```python
from build123d import *

# Parameters (mm, degrees)
SKETCH1_W               = 50
SKETCH1_H               = 50
BOSS_EXTRUDE1_DEPTH     = 2
SKETCH2_W               = 8.5
SKETCH2_H               = 2
SKETCH2_W_2             = 26.5
BOSS_EXTRUDE2_DEPTH     = 20
SKETCH3_W               = 2
SKETCH3_H               = 15
BOSS_EXTRUDE3_DEPTH     = 15
SKETCH5_W               = 2
SKETCH5_H               = 15
BOSS_EXTRUDE5_DEPTH     = 25
SKETCH6_W               = 8
SKETCH6_H               = 5
SKETCH6_H_2             = 10
BOSS_EXTRUDE6_DEPTH     = 2
FILLET1_R               = 10
FILLET2_R               = 10
FILLET3_R               = 5
CUT_EXTRUDE1_DEPTH      = 58.567351858
CUT_EXTRUDE1_DEPTH_BACK = 58.567351858
SKETCH7_R               = 1.65
SKETCH8_W               = 3.5
SKETCH8_H               = 6
BOSS_EXTRUDE7_DEPTH     = 8


with BuildPart() as part:
    # Sketch1 → Boss-Extrude1 (new body)
    with BuildSketch(Plane.XY):
        Rectangle(SKETCH1_W, SKETCH1_H)
    extrude(amount=BOSS_EXTRUDE1_DEPTH)

    # Sketch2 → Boss-Extrude2 (add)
    with BuildSketch(Plane(origin=(0, 0, 0), x_dir=(-1, 0, 0), z_dir=(0, 0, -1))):
        with Locations((-20.75, -24)):
            Rectangle(SKETCH2_W, SKETCH2_H)
        with Locations((11.75, -24)):
            Rectangle(SKETCH2_W_2, SKETCH2_H)
    extrude(amount=BOSS_EXTRUDE2_DEPTH)

    # Sketch3 → Boss-Extrude3 (add)
    with BuildSketch(Plane.XZ.offset(25)):
        with Locations((24, -5.5)):
            Rectangle(SKETCH3_W, SKETCH3_H)
    extrude(amount=BOSS_EXTRUDE3_DEPTH)

    # Sketch5 → Boss-Extrude5 (add)
    with BuildSketch(Plane(origin=(0, 0, 0), x_dir=(-1, 0, 0), z_dir=(0, 0, -1))):
        with Locations((-20.5, 5.5)):
            Rectangle(SKETCH5_W, SKETCH5_H)
        with Locations((22, 5.5)):
            Rectangle(SKETCH5_W, SKETCH5_H)
    extrude(amount=BOSS_EXTRUDE5_DEPTH)

    # Sketch6 → Boss-Extrude6 (add)
    with BuildSketch(Plane(origin=(0, 0, 0), x_dir=(-1, 0, 0), z_dir=(0, 0, -1))):
        with Locations((-29, -14)):
            Rectangle(SKETCH6_W, SKETCH6_H)
        with Locations((-29, 26)):
            Rectangle(SKETCH6_W, SKETCH6_H_2)
    extrude(amount=-BOSS_EXTRUDE6_DEPTH)

    # Fillet1
    # the kernel refuses this fillet: 10 mm, written as the material it adds along each edge
    with BuildSketch(Plane(origin=(25, 25, 0), x_dir=(-1, 0, 0), z_dir=(0, 0, 1))) as fillet1_piece_1:
        with BuildLine():
            CenterArc((9.16515139, -10), FILLET1_R, 90, 66.421821522)
            Line((0, -6), (-0.183303028, -5.92))
            ThreePointArc((-0.183303028, -5.92), (-0.2, -3), (-0.2, 0))
            Line((-0.2, 0), (0, 0.2))
            Line((0, 0.2), (9.16515139, 0.2))
            Line((9.16515139, 0.2), (9.16515139, 0))
        make_face()
    extrude(amount=2)

    # Fillet2
    # the kernel refuses this fillet: 10 mm, written as the material it adds along each edge
    with BuildSketch(Plane(origin=(25, 21, 0), x_dir=(0, -1, 0), z_dir=(0, 0, 1))) as fillet2_piece_1:
        with BuildLine():
            CenterArc((9.797958971, 10), FILLET2_R, 191.536959033, 78.463040967)
            Line((0, 8), (-0.195959179, 7.96))
            ThreePointArc((-0.195959179, 7.96), (-0.2, 4), (-0.2, 0))
            Line((-0.2, 0), (0, -0.2))
            Line((0, -0.2), (9.797958971, -0.2))
            Line((9.797958971, -0.2), (9.797958971, 0))
        make_face()
    extrude(amount=2)

    # Fillet3
    fillet3_edges = [part.edges().sort_by_distance(p)[0] for p in [
        (25, -16.5, 1),
        (25, -11.5, 1),
    ]]
    fillet(fillet3_edges, radius=FILLET3_R)

    # Sketch7 → Cut-Extrude1 (cut, two sides: drawn at the far end of the back side and taken through both)
    with BuildSketch(Plane(origin=(0, 0, 0), x_dir=(-1, 0, 0), z_dir=(0, 0, -1)).offset(-CUT_EXTRUDE1_DEPTH_BACK)):
        with Locations((-29.35, -14)):
            Circle(SKETCH7_R)
        with Locations((-29.35, 26)):
            Circle(SKETCH7_R)
    extrude(amount=CUT_EXTRUDE1_DEPTH + CUT_EXTRUDE1_DEPTH_BACK, mode=Mode.SUBTRACT)

    # Sketch8 → Boss-Extrude7 (add)
    with BuildSketch(Plane(origin=(0, 0, 0), x_dir=(-1, 0, 0), z_dir=(0, 0, -1))):
        with Locations((23.25, -11)):
            Rectangle(SKETCH8_W, SKETCH8_H)
    extrude(amount=BOSS_EXTRUDE7_DEPTH)


solid = part.part
```
Read the model definition and answer for the solid it produces. Units are mm, in the model's axes. A direction names the side the tool comes from. Coordinates: 2 decimals unless noted, no trailing zeros. Write each loop counter-clockwise with the first axis right and the second up, starting at its lowest first coordinate (ties: lowest second). Pieces come first, ordered by that corner, then holes. Notation, with made-up numbers: (28, 21.25) -> (71, 21.25) arc R28 cw to (71, 52.25) -> close; hole circle Ø9 at (-33.5, 81.25). An arc over 180 degrees is marked (long way). Return JSON: item names as keys, results as strings.
1. A cutting plane is placed at C-C (z = -4.5). Determine the outline of the cut face in (x, y), and give its area (3 significant figures).
Found:
{"outline": "(-25, -25) -> (1.5, -25) -> (1.5, -23) -> (-25, -23) -> close; (-25, -14) -> (-21.5, -14) -> (-21.5, -8) -> (-25, -8) -> close; (-23, -2) -> (-21, -2) -> (-21, 13) -> (-23, 13) -> close; (16.5, -25) -> (23, -25) -> (23, -40) -> (25, -40) -> (25, -23) -> (16.5, -23) -> close; (19.5, -2) -> (21.5, -2) -> (21.5, 13) -> (19.5, 13) -> close", "area": "181 mm2"}
2. A cutting plane is placed at D-D (y = 26). Determine the outline of the cut face in (x, z), and give its area (3 significant figures).
Found:
{"outline": "(20.19, 0) -> (27.7, 0) -> (27.7, 2) -> (20.19, 2) -> close; (31, 0) -> (33, 0) -> (33, 2) -> (31, 2) -> close", "area": "19.0 mm2"}
3. Determine the mould class of faces 1 (the face through (25, -31, -7)), 2 (the face through (21, -2, -12)), 3 (the face through (-22, 13, -12)) for opening direction Y: pulls with the +Y half, pulls with the -Y half, needs draft (parallel to the pull), parting line crosses it, or undercut.
Found:
{"face 1": "needs draft", "face 2": "undercut", "face 3": "pulls with the +Y half"}
4. A cutting plane is placed at A-A (z = -11.5). Determine the outline of the cut face in (x, y), and give its area (3 significant figures).
Found:
{"outline": "(-25, -25) -> (1.5, -25) -> (1.5, -23) -> (-25, -23) -> close; (-23, -2) -> (-21, -2) -> (-21, 13) -> (-23, 13) -> close; (16.5, -25) -> (23, -25) -> (23, -40) -> (25, -40) -> (25, -23) -> (16.5, -23) -> close; (19.5, -2) -> (21.5, -2) -> (21.5, 13) -> (19.5, 13) -> close", "area": "160 mm2"}
5. Find the intervals of material crossed by line 1 along Y through (x, z) = (29.35, 0.75); line 2 along X through (y, z) = (-14, 1.45); line 3 along Z through (x, y) = (-18, 12), in increasing order. Write a range as from..to.
Found:
{"line 1": "-16.54..-15.65, -12.35..-11.46, 19.45..24.35, 27.65..31", "line 2": "-25..27.7, 31..33", "line 3": "0..2"}
6. A tool of negligible diameter and unlimited length cuts with its end or side. For faces 4 (the face through (-23, 5, -12)), 5 (the face through (25, 2, 1)), 6 (the face through (-21, 5, -12)), 7 (the face through (-22, -2, -12)), from which of +Z, -Z, +X, -X, +Y, -Y can it reach the whole face along a straight path? Write none if from no direction.
Found:
{"face 4": "-Z, -X, +Y", "face 5": "+Z, -Z, +X", "face 6": "-Z, +Y", "face 7": "-Z, +X, -X"}
7. A cutting plane is placed at B-B (z = -21.5). Determine the outline of the cut face in (x, y).
Found:
{"outline": "(-23, -2) -> (-21, -2) -> (-21, 13) -> (-23, 13) -> close; (19.5, -2) -> (21.5, -2) -> (21.5, 13) -> (19.5, 13) -> close"}
8. Each of these flat-tipped pins is pushed along its axis until it touches: P1, Ø6, axis at x = -5.5, z = -9, coming from the +Y side; P2, Ø2, axis at x = -8.5, y = -23.5, coming from the -Z side; P3, Ø4, axis at x = -14.5, z = -3, coming from the -Y side; P4, Ø3, axis at x = 29.35, y = -14, coming from the -Z side. Where does it stop, or does it pass through?
Found:
{"P1": "y = -23", "P2": "z = -20", "P3": "y = -25", "P4": "through"}
